Can you work these out from the drawing? Everything is in mm from the part's minimum corner. A direction names the side the tool comes from. Round coordinates to 2 decimals unless told otherwise and drop trailing zeros. Loops run counter-clockwise (first coordinate to the right, second up) from the corner with the lowest first, then second, coordinate; pieces in that order, holes last. Notation, with made-up numbers: M 27,-31.5 L 64,-31.5 A10 cw 64,-19.5 Z; hole C 77,66 d2. An arc over 180 degrees is marked long. Use a Markdown table: item, result.
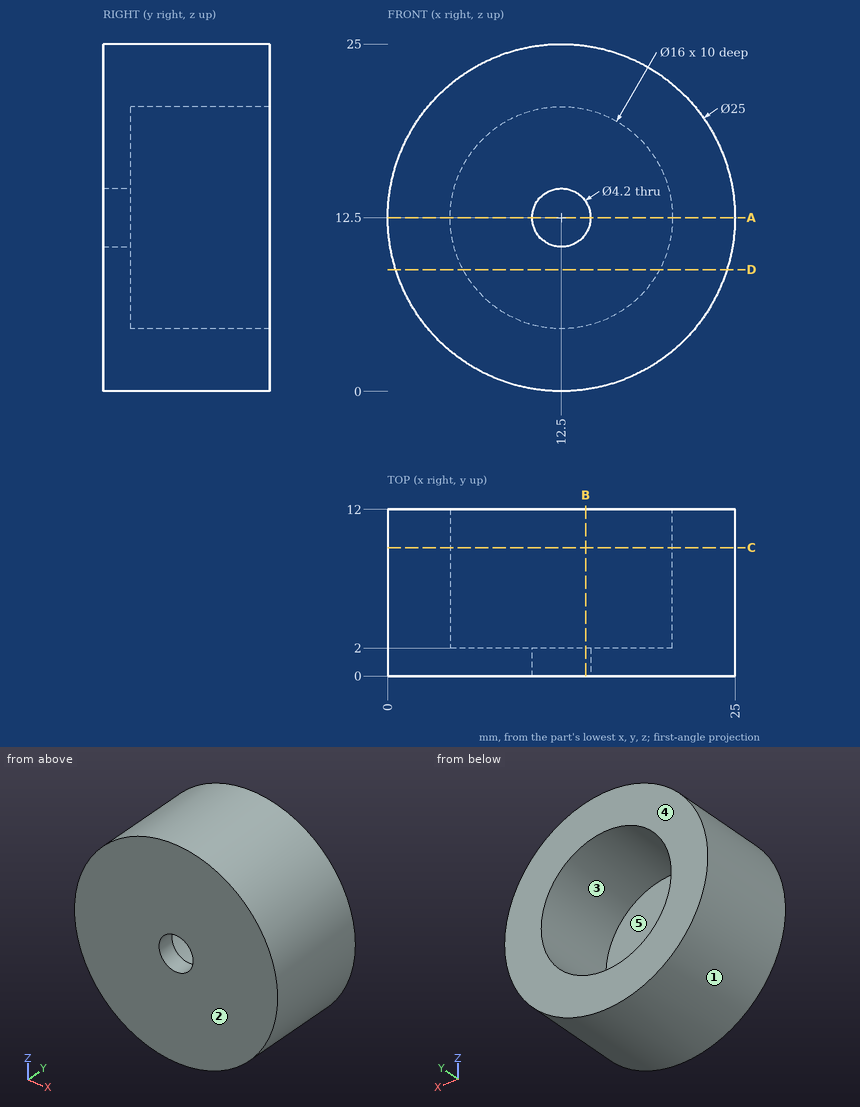
Q1. I need wall thicknesses on line 1 (X direction, y = 0.65, z = 12.5); line 2 (Z direction, x = 12.5, y = 9). Which ranges of each line are inside material? Lowest first, please. Write a range as from..to.
Return value:
| item | result |
|---|---|
| line 1 | x = 0..10.4, 14.6..25 |
| line 2 | z = 0..4.5, 20.5..25 |
Q2. Imagine slicing it at C-C, the plane y = 9.25. Please give me the cut outline in (x, z).
Return value:
| item | result |
|---|---|
| outline | C 12.5,12.5 d25; hole C 12.5,12.5 d16 |
Q3. Imagine slicing it at A-A, the plane z = 12.5. Please give me the cut outline in (x, y).
Return value:
| item | result |
|---|---|
| outline | M 0,0 L 10.4,0 L 10.4,2 L 4.5,2 L 4.5,12 L 0,12 Z; M 14.6,0 L 25,0 L 25,12 L 20.5,12 L 20.5,2 L 14.6,2 Z |
Q4. Imagine slicing it at D-D, the plane z = 8.75. Please give me the cut outline in (x, y).
Return value:
| item | result |
|---|---|
| outline | M 0.58,0 L 24.42,0 L 24.42,12 L 19.57,12 L 19.57,2 L 5.43,2 L 5.43,12 L 0.58,12 Z |
Q5. For the marked faces 4 and 5, which set-ups out of +Z, -Z, +X, -X, +Y, -Y let a thin tool reach every point of the face, with its end or its side?
Return value:
| item | result |
|---|---|
| face 4 | +Z, -Z, +X, -X, +Y |
| face 5 | +Y |
Q6. We'd pull the mould along Z, two halves only. Please class the marked faces 1, 2 and 3: pulls with the +Z half, pulls with the -Z half, needs draft (parallel to the pull), parting line crosses it, or undercut.
Return value:
| item | result |
|---|---|
| face 1 | parting line crosses it |
| face 2 | needs draft |
| face 3 | undercut |
Q7. Will these pins go through, and if not, where does the flat tip stop? P1, Ø5, axis at x = 12.5, z = 12.5, coming from the +Y side; P2, Ø3, axis at x = 14.5, y = 6.5, coming from the -Z side.
Return value:
| item | result |
|---|---|
| P1 | stops at y = 2 |
| P2 | stops at z = 0.01 |
Q8. Imagine slicing it at B-B, the plane x = 14.25. Please give me the cut outline in (y, z), then the cut area to 3 significant figures.
Return value:
| item | result |
|---|---|
| outline | M 0,0.12 L 12,0.12 L 12,4.69 L 2,4.69 L 2,11.34 L 0,11.34 Z; M 0,13.66 L 2,13.66 L 2,20.31 L 12,20.31 L 12,24.88 L 0,24.88 Z |
| area | 136 mm^2 |
